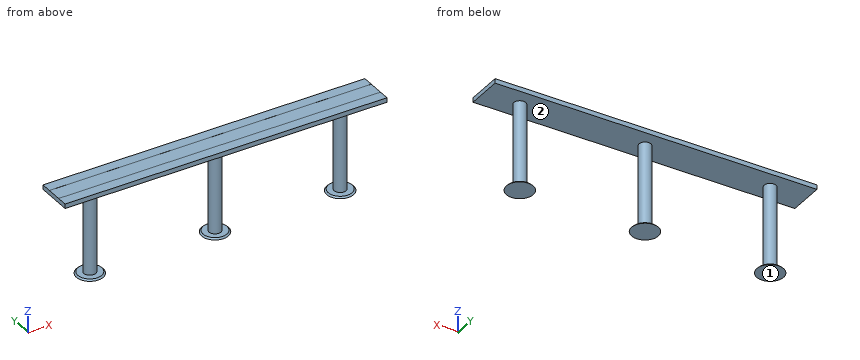
```python
from build123d import *

# Parameters (mm, degrees)
F0_W     = 2743.2
F0_H     = 304.8
F1_DEPTH = 38.1
F2_R     = 50.8
F3_DEPTH = 736.6
F4_R     = 114.3
F5_DEPTH = 12.7
F5_TAPER = 45
F6_W     = 2743.2
F6_H     = 88.9
F7_DEPTH = 0.3175


with BuildPart() as f1:
    # F0 (on Top) → F1 (new body)
    with BuildSketch(Plane.XY):
        Rectangle(F0_W, F0_H)
    extrude(amount=F1_DEPTH)

    # F2 (on face) → F3 (join)
    with BuildSketch(Plane(origin=(0, 0, 0), x_dir=(1, 0, 0), z_dir=(0, 0, -1))):
        with Locations((-1066.8, 0)):
            Circle(F2_R)
        with Locations((1066.8, 0)):
            Circle(F2_R)
        Circle(F2_R)
    extrude(amount=F3_DEPTH)

    # F4 (on face) → F5 (join)
    with BuildSketch(Plane(origin=(0, 0, -736.6), x_dir=(1, 0, 0), z_dir=(0, 0, -1))):
        with Locations((-1066.8, 0)):
            Circle(F4_R)
        with Locations((1066.8, 0)):
            Circle(F4_R)
        Circle(F4_R)
    extrude(amount=-F5_DEPTH, taper=F5_TAPER)

    # F6 (on face) → F7 (join)
    with BuildSketch(Plane.XY.offset(38.1)):
        with Locations((0, 107.95)):
            Rectangle(F6_W, F6_H)
        with Locations((0, -107.95)):
            Rectangle(F6_W, F6_H)
    extrude(amount=F7_DEPTH)


solid = f1.part
```
Here's how the part is built. I have some questions about the finished solid (model axes, mm). Face numbers are marked on the shaded views. Round coordinates to 2 decimals unless told otherwise and drop trailing zeros. Order: outer loops, then holes, each group sorted by start corner. A loop starts at its lowest first (then second) coordinate and runs counter-clockwise, first axis right, second up. Notation, with made-up numbers: (-18, 53) -> (5, 53) arc R19 cw to (5, 76) -> close; hole circle Ø2 at (62, -18). An arc over 180 degrees is marked (long way). Use a Markdown table: item, result. Add a question column.
(1) For pin 1 Ø2 at (y, z) = (-41.5, -144) entering from -X; pin 2 Ø1.5 at (x, y) = (-935.5, -40) entering from -Z; pin 3 Ø2 at (y, z) = (-8.5, -360) entering from -X, each with a flat end and sliding along its axis, tell me the tip position at first contact or that it passes through.
(2) Suppose I cut it at B-B, the plane x = -912. Please give me the cut outline in (y, z).
(3) If we mould it in two halves opening along X, with no side actions, what happens to the marked faces 1 and 2? For each: released by +X, released by -X, zero draft, split by the parting line, or undercut.
(4) I need wall thicknesses on line 1 along X through (y, z) = (-6.5, -128.5); line 2 along X through (y, z) = (1, -476.5); line 3 along Z through (x, y) = (-1143.5, -35.5). Which ranges of each line are inside material? Lowest first, please.
(5) Suppose I cut it at A-A, the plane z = -220. Please give me the cut outline in (x, y).
Verdict:
| question | item | result |
|---|---|---|
| 1 | pin 1 | x = -1097.47 |
| 1 | pin 2 | z = 0 |
| 1 | pin 3 | x = -1117.04 |
| 2 | outline | (-152.4, 0) -> (152.4, 0) -> (152.4, 38.42) -> (63.5, 38.42) -> (63.5, 38.1) -> (-63.5, 38.1) -> (-63.5, 38.42) -> (-152.4, 38.42) -> close |
| 3 | face 1 | zero draft |
| 3 | face 2 | undercut |
| 4 | line 1 | -1117.18 to -1016.42, -50.38 to 50.38, 1016.42 to 1117.18 |
| 4 | line 2 | -1117.59 to -1016.01, -50.79 to 50.79, 1016.01 to 1117.59 |
| 4 | line 3 | -736.6 to -723.9, 0 to 38.1 |
| 5 | outline | circle Ø101.6 at (-1066.8, 0); circle Ø101.6 at (0, 0); circle Ø101.6 at (1066.8, 0) |
